```python
from build123d import *

# Parameters (mm, degrees)
F0_R     = 0.325
F0_W     = 0.54
F0_H     = 1.2
F1_DEPTH = 2.5


with BuildPart() as f1:
    # F0 (on Top) → F1 (new body)
    with BuildSketch(Plane.XY):
        Polygon((-71.271986, 0), (-69.271986, 0), (-69.271986, 0.4), (-69.271986, 1.6), (-69.271986, 2), (-71.271986, 2), align=None)
        with Locations((-70.271986, 1)):
            Circle(F0_R, mode=Mode.SUBTRACT)
        with Locations((-69.001986, 1)):
            Rectangle(F0_W, F0_H)
        Polygon((-68.731986, 1.6), (-68.731986, 0.4), (-68.731986, 0), (-66.731986, 0), (-66.731986, 0.4), (-66.731986, 1.6), (-66.731986, 2), (-68.731986, 2), align=None)
        with Locations((-67.731986, 1)):
            Circle(F0_R, mode=Mode.SUBTRACT)
        with Locations((-66.461986, 1)):
            Rectangle(F0_W, F0_H)
        Polygon((-66.191986, 1.6), (-66.191986, 0.4), (-66.191986, 0), (-64.191986, 0), (-64.191986, 0.4), (-64.191986, 1.6), (-64.191986, 2), (-66.191986, 2), align=None)
        with Locations((-65.191986, 1)):
            Circle(F0_R, mode=Mode.SUBTRACT)
        with Locations((-63.921986, 1)):
            Rectangle(F0_W, F0_H)
        Polygon((-63.651986, 1.6), (-63.651986, 0.4), (-63.651986, 0), (-61.651986, 0), (-61.651986, 0.4), (-61.651986, 1.6), (-61.651986, 2), (-63.651986, 2), align=None)
        with Locations((-62.651986, 1)):
            Circle(F0_R, mode=Mode.SUBTRACT)
    extrude(amount=F1_DEPTH)


solid = f1.part
```
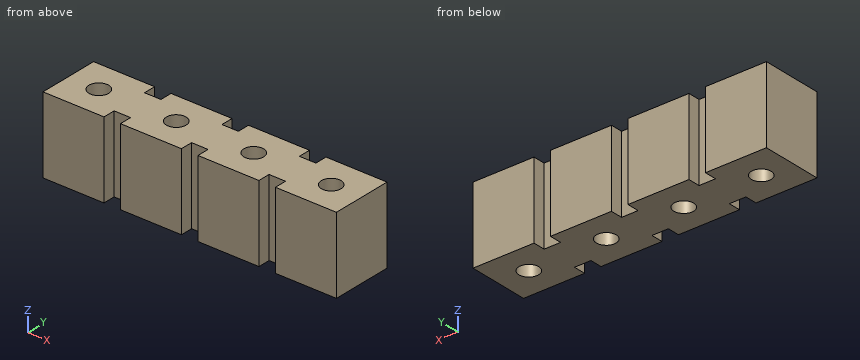
Check sheet for the modelled part. Datum: model origin and axes. Units: mm. Give positions to 0.01 mm unless a question says otherwise; leave off trailing zeros. Order: outer loops, then holes, each group sorted by start corner. A loop starts at its lowest first (then second) coordinate and runs counter-clockwise, first axis right, second up. Notation, with made-up numbers: (27.5, -22.75) -> (78.5, -22.75) arc R16 cw to (78.5, -18.75) -> close; hole circle Ø1 at (64.25, 50). An arc over 180 degrees is marked (long way). Return JSON: item names as keys, results as strings.
1. Cross-section at A-A, the plane y = 1. Record the cut outline in (x, z), plus the area to 4 significant figures.
From the geometry:
{"outline": "(-71.27, 0) -> (-70.6, 0) -> (-70.6, 2.5) -> (-71.27, 2.5) -> close; (-69.95, 0) -> (-68.06, 0) -> (-68.06, 2.5) -> (-69.95, 2.5) -> close; (-67.41, 0) -> (-65.52, 0) -> (-65.52, 2.5) -> (-67.41, 2.5) -> close; (-64.87, 0) -> (-62.98, 0) -> (-62.98, 2.5) -> (-64.87, 2.5) -> close; (-62.33, 0) -> (-61.65, 0) -> (-61.65, 2.5) -> (-62.33, 2.5) -> close", "area": "17.55 mm^2"}
2. Material ranges on probe 1 along X at (y, z) = (1.05, 1.6); probe 2 along Y at (x, z) = (-64, 0.3), recorded low to high. Write a range as [from, to].
From the geometry:
{"probe 1": "[-71.27, -70.59], [-69.95, -68.05], [-67.41, -65.51], [-64.87, -62.97], [-62.33, -61.65]", "probe 2": "[0.4, 1.6]"}
3. Cross-section at C-C, the plane x = -70.5. Record the cut outline in (y, z).
From the geometry:
{"outline": "(0, 0) -> (0.77, 0) -> (0.77, 2.5) -> (0, 2.5) -> close; (1.23, 0) -> (2, 0) -> (2, 2.5) -> (1.23, 2.5) -> close"}
4. Cross-section at D-D, the plane x = -62.75. Record the cut outline in (y, z).
From the geometry:
{"outline": "(0, 0) -> (0.69, 0) -> (0.69, 2.5) -> (0, 2.5) -> close; (1.31, 0) -> (2, 0) -> (2, 2.5) -> (1.31, 2.5) -> close"}
5. Cross-section at B-B, the plane z = 2.15. Count the separate pieces of the cut face and the enclosed holes in it, plus the area to 3 significant figures.
From the geometry:
{"separate pieces": "1", "enclosed holes": "4", "area": "16.6 mm^2"}
